Could you check a few things on this model? Use its own coordinates, in mm. Give positions to 0.01 mm unless a question says otherwise; leave off trailing zeros. Write each loop counter-clockwise with the first axis right and the second up, starting at its lowest first coordinate (ties: lowest second). Pieces come first, ordered by that corner, then holes. Notation, with made-up numbers: (74.5, 19) -> (122.5, 19) arc R9 cw to (122.5, 30) -> close; hole circle Ø10 at (6.25, -29). An arc over 180 degrees is marked (long way). Write item = value, one per line. Start each with the question number.
```python
from build123d import *

# Parameters (mm, degrees)
SKETCH1_W               = 304.8
SKETCH1_H               = 304.8
BOSS_EXTRUDE1_DEPTH     = 10.16
CUT_EXTRUDE1_DEPTH      = 223.167807436
CUT_EXTRUDE1_DEPTH_BACK = 223.167807436
SKETCH2_R               = 3.04
SKETCH4_R               = 3.2281005
CUT_EXTRUDE3_DEPTH      = 345.170558112
CUT_EXTRUDE4_DEPTH      = 345.170558112
CUT_EXTRUDE4_DEPTH_BACK = 345.170558112
SKETCH5_R               = 3.308101134
CUT_EXTRUDE5_DEPTH      = 345.170558112
CUT_EXTRUDE5_DEPTH_BACK = 345.170558112
SKETCH3_R               = 3
SKETCH6_R               = 2.704571709
CUT_EXTRUDE6_DEPTH      = 345.170558112


with BuildPart() as part:
    # Sketch1 → Boss-Extrude1 (new body)
    with BuildSketch(Plane(origin=(0, 0, 0), x_dir=(1, 0, 0), z_dir=(0, 1, 0))):
        with Locations((-7.121495327, 1.899065421)):
            Rectangle(SKETCH1_W, SKETCH1_H)
    extrude(amount=BOSS_EXTRUDE1_DEPTH)

    # Sketch2 → Cut-Extrude1 (cut, two sides: drawn at the far end of the back side and taken through both)
    with BuildSketch(Plane.XY.offset(-CUT_EXTRUDE1_DEPTH_BACK)):
        with Locations((-7.121495327, 4.941750029)):
            Circle(SKETCH2_R)
    extrude(amount=CUT_EXTRUDE1_DEPTH + CUT_EXTRUDE1_DEPTH_BACK, mode=Mode.SUBTRACT)

    # Sketch4 → Cut-Extrude3 (cut, through all)
    with BuildSketch(Plane.XY.offset(150.500934579)):
        with Locations((-87.118814918, 5.218403667)):
            Circle(SKETCH4_R)
    extrude(amount=-CUT_EXTRUDE3_DEPTH, mode=Mode.SUBTRACT)

    # Sketch5 → Cut-Extrude4 (cut, two sides: drawn at the far end of the back side and taken through both)
    with BuildSketch(Plane.XY.offset(150.500934579).offset(-CUT_EXTRUDE4_DEPTH_BACK)):
        with Locations((-33.586304402, 5.334469318)):
            Circle(SKETCH5_R)
    extrude(amount=CUT_EXTRUDE4_DEPTH + CUT_EXTRUDE4_DEPTH_BACK, mode=Mode.SUBTRACT)

    # Sketch3 → Cut-Extrude5 (cut, two sides: drawn at the far end of the back side and taken through both)
    with BuildSketch(Plane.XY.offset(150.500934579).offset(-CUT_EXTRUDE5_DEPTH_BACK)):
        with Locations((-54.67948523, 4.941750029)):
            Circle(SKETCH3_R)
    extrude(amount=CUT_EXTRUDE5_DEPTH + CUT_EXTRUDE5_DEPTH_BACK, mode=Mode.SUBTRACT)

    # Sketch6 → Cut-Extrude6 (cut, through all)
    with BuildSketch(Plane.XY.offset(150.500934579)):
        with Locations((-96.021495327, 5.218403667)):
            Circle(SKETCH6_R)
    extrude(amount=-CUT_EXTRUDE6_DEPTH, mode=Mode.SUBTRACT)


solid = part.part
```
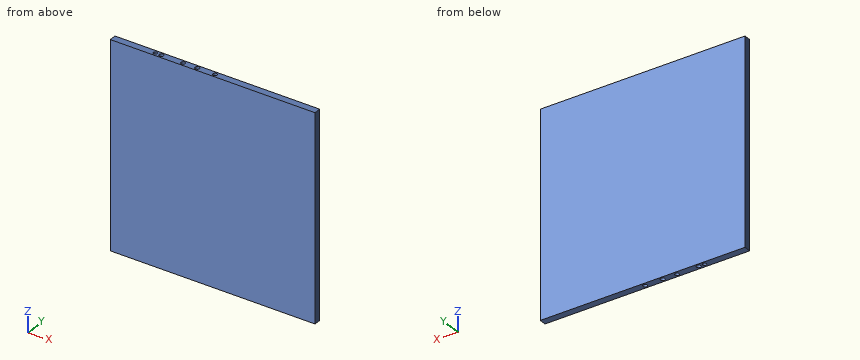
(1) If I drill on line 1 along X through (y, z) = (4.75, 68.5); line 2 along X through (y, z) = (5.25, 90.5); line 3 along Y through (x, z) = (-89, 35), over which ranges is the centre line in solid material (lowest first)? Write a range as from..to.
(2) I'm going to push a flat-ended pin straight in: pin 1 (6 mm diameter, centred on x = -33.59, y = 5.33, fed in from -Z). Where does the tip first touch, or does it pass through?
(3) Imagine slicing it at A-A (z = 7). Please give me the cut outline in (x, y), then the cut area to 3 significant figures.
Answers below:
q1.line_1 = -159.52..-98.69, -93.36..-90.31, -83.92..-57.67, -51.69..-36.84, -30.33..-10.16, -4.09..145.28
q1.line_2 = -159.52..-98.73, -93.32..-90.35, -83.89..-57.66, -51.7..-36.89, -30.28..-10.15, -4.1..145.28
q1.line_3 = 0..2.6, 7.84..10.16
q2.pin_1 = through
q3.outline = (-159.52, 0) -> (145.28, 0) -> (145.28, 10.16) -> (-159.52, 10.16) -> close; hole circle Ø5.41 at (-96.02, 5.22); hole circle Ø6.46 at (-87.12, 5.22); hole circle Ø6 at (-54.68, 4.94); hole circle Ø6.62 at (-33.59, 5.33); hole circle Ø6.08 at (-7.12, 4.94)
q3.area = 2,950 mm^2
